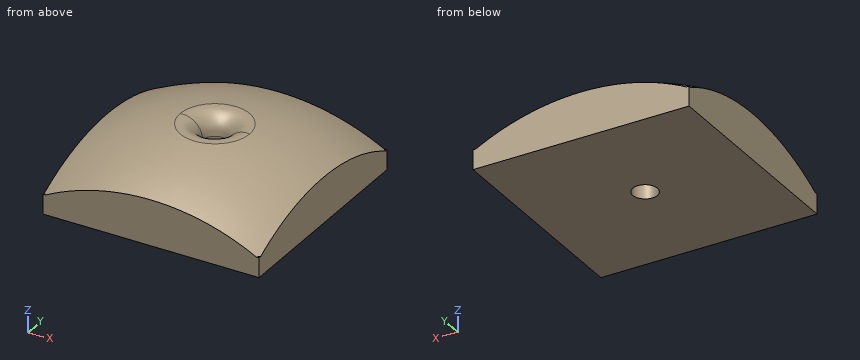
```python
from build123d import *

# Parameters (mm, degrees)
F0_W     = 139.7
F0_H     = 139.7
F0_R     = 7.9375
F1_DEPTH = 12.7
F4_W     = 59.6992075443
F4_H     = 63.3541112766
F4_W_2   = 56.6389337182
F4_H_2   = 62.1770434082
F5_DEPTH = 101.6
F6_W     = 47.2303777933
F6_H     = 39.3290324137
F6_W_2   = 46.0887253284
F6_H_2   = 41.5412890725
F7_DEPTH = 101.6
F9_DEPTH = 76.2
F10_R    = 12.7


# Not quite as in the source:
# - a feature names something its author has since deleted; it is built from what else it names


with BuildPart() as f1:
    # F0 (on Top) → F1 (new body)
    with BuildSketch(Plane.XY):
        Rectangle(F0_W, F0_H)
        Circle(F0_R, mode=Mode.SUBTRACT)
    extrude(amount=F1_DEPTH)

    # F2 (on Front) → F3 (revolve)
    with BuildSketch(Plane.XZ):
        with BuildLine():
            Line((0, 0), (0, 45.1088836892))
            ThreePointArc((0, 45.1088836892), (-60.5414406288, 33.4106062222), (-112.3665997793, 0))
            Line((-112.3665997793, 0), (0, 0))
        make_face()
    revolve(axis=Axis((0, 0, 22.5544418446), (0, 0, -1)))

    # F4 (on Front) → F5 (cut, symmetric)
    with BuildSketch(Plane.XZ):
        with Locations((-99.4039475918, 19.7528828867)):
            Rectangle(F4_W, F4_H)
        with Locations((97.9946739972, 18.4055566788)):
            Rectangle(F4_W_2, F4_H_2)
    extrude(amount=F5_DEPTH, both=True, mode=Mode.SUBTRACT)

    # F6 (on Right) → F7 (cut, symmetric)
    with BuildSketch(Plane.YZ):
        with Locations((-93.4242233634, 10.9358266927)):
            Rectangle(F6_W, F6_H)
        with Locations((92.853397131, 9.8296983633)):
            Rectangle(F6_W_2, F6_H_2)
    extrude(amount=F7_DEPTH, both=True, mode=Mode.SUBTRACT)

    # F0 (on Top) → F9 (cut, symmetric)
    with BuildSketch(Plane.XY):
        Circle(F0_R)
    extrude(amount=F9_DEPTH, both=True, mode=Mode.SUBTRACT)

    # F10
    f10_edges = [f1.edges().sort_by_distance(p)[0] for p in [
        (0, -7.9375, 44.914919),
        (0, 7.9375, 44.914919),
    ]]
    fillet(f10_edges, radius=F10_R)


solid = f1.part
```
For this review, take the finished solid that the model builds, in its own axes (mm). Round coordinates to 2 decimals unless told otherwise and drop trailing zeros. Write each loop counter-clockwise with the first axis right and the second up, starting at its lowest first coordinate (ties: lowest second). Pieces come first, ordered by that corner, then holes. Notation, with made-up numbers: (14, -34.5) -> (55, -34.5) arc R21 cw to (55, -22.5) -> close; hole circle Ø7 at (18.5, 22.5). An arc over 180 degrees is marked (long way). One line per question, with ' | ' between items. Start each with the question number.
(1) Insertion check: P1, Ø1.8, axis at x = -69, y = -68.5, coming from the +Z side; P2, Ø1, axis at x = -36.5, y = 55, coming from the -Z side; P3, Ø0.5, axis at x = -69, y = 69, coming from the +Z side; P4, Ø20.5, axis at x = 0, y = 0, coming from the +Z side. Each pin has a flat end and moves straight along its axis. Give the tip position at first contact, or say it passes through.
(2) Add section B-B, the plane y = 55. Write out the cut boundary in (x, z), plus the area to 3 significant figures.
(3) Add section A-A, the plane z = 17. Write out the cut boundary in (x, y) (1 decimal), plus the area to 3 significant figures.
(4) Add section C-C, the plane x = -48. Write out the cut boundary in (y, z), plus the area to 3 significant figures.
(5) For line 1 along Y through (x, z) = (0, 8); line 2 along X through (y, z) = (-0.5, 12); line 3 along X through (y, z) = (27.5, 29), list the stretches that pass through material, from the lowest coordinate up. Write a range as from..to.
Answer list:
1) P1: z = 13.48 | P2: z = 0 | P3: z = 12.74 | P4: z = 38.29
2) outline: (-69.55, 0) -> (69.68, 0) -> (69.68, 18.72) arc R152.92 ccw to (-69.55, 18.78) -> close | area: 4,190 mm²
3) outline: (-69.6, -59.2) arc R91.4 ccw to (-58.9, -69.8) -> (58.9, -69.8) arc R91.4 ccw to (69.7, -59.1) -> (69.7, 59.1) arc R91.4 ccw to (58.9, 69.8) -> (-58.9, 69.8) arc R91.4 ccw to (-69.6, 59.2) -> close; hole circle Ø15.9 at (0, 0) | area: 19,000 mm²
4) outline: (-69.81, 0) -> (69.81, 0) -> (69.81, 21.28) arc R155.26 ccw to (-69.81, 21.28) -> close | area: 4,530 mm²
5) line 1: -69.81..-7.94, 7.94..69.81 | line 2: -69.55..-7.92, 7.92..69.68 | line 3: -64.96..64.96
